from build123d import *

# Parameters (mm, degrees)
SKETCH_1_W          = 10
SKETCH_1_H          = 55.540767131
EXTRUDE_1_DEPTH     = 25
SKETCH_5_R          = 4.000000001
CUT_EXTRUDE_2_DEPTH = 74.509784895
CUT_EXTRUDE_3_DEPTH = 74.509784895
CHAMFER_1_SIZE      = 4


with BuildPart() as part:
    # Эскиз1 → Вытянуть1 (new body)
    with BuildSketch(Plane(origin=(0, 0, 0), x_dir=(0, 0, -1), z_dir=(1, 0, 0))):
        with Locations((-15, -40.630555576)):
            Rectangle(SKETCH_1_W, SKETCH_1_H)
    extrude(amount=EXTRUDE_1_DEPTH)

    # Эскиз5 → Вырез-Вытянуть2 (cut, through all)
    with BuildSketch(Plane.XY.offset(20)):
        with Locations((15, -40.630555576)):
            Circle(SKETCH_5_R)
    extrude(amount=-CUT_EXTRUDE_2_DEPTH, mode=Mode.SUBTRACT)

    # Эскиз6 → Вырез-Вытянуть3 (cut, through all)
    with BuildSketch(Plane.XY.offset(20)):
        Polygon((22.828613207, -50.630555576), (22.828613207, -30.630555576), (8.828613207, -30.630555576), (8.828613207, -12.86017201), (25, -12.86017201), (25, -68.400939141), (8.828613207, -68.400939141), (8.828613207, -50.630555576), align=None)
    extrude(amount=-CUT_EXTRUDE_3_DEPTH, mode=Mode.SUBTRACT)

    # Фаска1
    chamfer_1_edges = [part.edges().sort_by_distance(p)[0] for p in [
        (22.828613207, -30.630555576, 15),
        (8.828613207, -12.86017201, 15),
        (8.828613207, -68.400939141, 15),
        (22.828613207, -50.630555576, 15),
    ]]
    chamfer(chamfer_1_edges, length=CHAMFER_1_SIZE)


solid = part.part
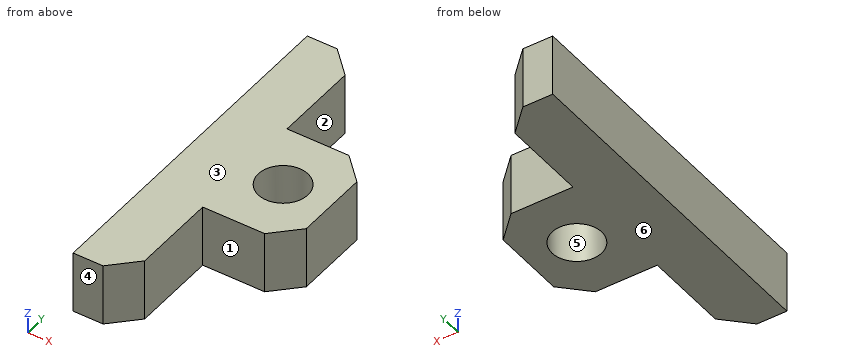
Part model, mm, in its own coordinate system. Face numbers are marked on the shaded views. A direction names the side the tool comes from. Round coordinates to 2 decimals unless told otherwise and drop trailing zeros. Order: outer loops, then holes, each group sorted by start corner. A loop starts at its lowest first (then second) coordinate and runs counter-clockwise, first axis right, second up. Notation, with made-up numbers: (3, -19) -> (22, -19) arc R22 ccw to (22, 17) -> close; hole circle Ø8 at (64, 42). An arc over 180 degrees is marked (long way). Put each result on its own line as item: value.
Q1. Band-saw the part on D-D (y = -49). Give the cut face in (x, z), and give its area (3 significant figures).
From the geometry:
outline: (0, 10) -> (20.46, 10) -> (20.46, 20) -> (0, 20) -> close
area: 205 mm2
Q2. Band-saw the part on C-C (x = 18.25). Give the cut face in (y, z), and give its area (3 significant figures).
From the geometry:
outline: (-50.63, 10) -> (-42.96, 10) -> (-42.96, 20) -> (-50.63, 20) -> close; (-38.3, 10) -> (-30.63, 10) -> (-30.63, 20) -> (-38.3, 20) -> close
area: 153 mm2
Q3. Band-saw the part on A-A (x = 15). Give the cut face in (y, z), and give its area (3 significant figures).
From the geometry:
outline: (-50.63, 10) -> (-44.63, 10) -> (-44.63, 20) -> (-50.63, 20) -> close; (-36.63, 10) -> (-30.63, 10) -> (-30.63, 20) -> (-36.63, 20) -> close
area: 120 mm2
Q4. Band-saw the part on B-B (z = 14). Give the cut face in (x, y).
From the geometry:
outline: (0, -68.4) -> (4.83, -68.4) -> (8.83, -64.4) -> (8.83, -50.63) -> (18.83, -50.63) -> (22.83, -46.63) -> (22.83, -34.63) -> (18.83, -30.63) -> (8.83, -30.63) -> (8.83, -16.86) -> (4.83, -12.86) -> (0, -12.86) -> close; hole circle Ø8 at (15, -40.63)
Q5. Pull direction Y, two halves, no side cores. Call the marked faces 4, 5 and 6: pulls with the +Y half, pulls with the -Y half, needs draft (parallel to the pull), parting line crosses it, or undercut.
From the geometry:
face 4: pulls with the -Y half
face 5: undercut
face 6: needs draft
Q6. Wall check: line 1 (Y direction, x = 15, z = 13.75); line 2 (X direction, y = -52, z = 12.5); line 3 (X direction, y = -42.5, z = 13.5). Give the ranges that are in metal, low to high. Write a range as [from, to].
From the geometry:
line 1: y = [-50.63, -44.63], [-36.63, -30.63]
line 2: x = [0, 8.83]
line 3: x = [0, 11.46], [18.54, 22.83]
Q7. Tool access for the marked faces 1, 2 and 3: list every direction of +Z, -Z, +X, -X, +Y, -Y with a clear straight run to the whole face (end or side of a thin tool).
From the geometry:
face 1: +Z, -Z, +X, -Y
face 2: +Z, -Z, +X, +Y
face 3: +Z, +X, -X, +Y, -Y
Q8. Pin check, flat tips, straight feed: pin 1 Ø3 at (y, z) = (-56.5, 17) entering from +X; pin 2 Ø5 at (x, z) = (14, 16) entering from -Y; pin 3 Ø6 at (x, z) = (15, 15) entering from +Y; pin 4 Ø12 at (x, y) = (12.5, -29) entering from -Z. Stop position of each tip, or through.
From the geometry:
pin 1: stops at x = 8.83
pin 2: stops at y = -50.63
pin 3: stops at y = -30.63
pin 4: stops at z = 10
